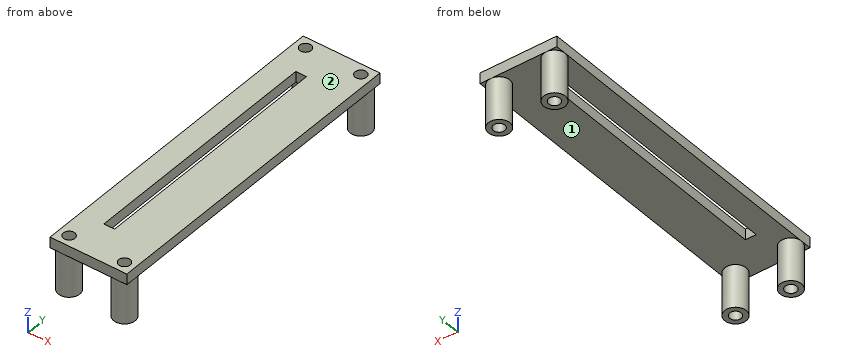
```python
from build123d import *

# Parameters (mm, degrees)
SKETCH1_W           = 21.5
SKETCH1_H           = 91
SKETCH1_R           = 1.6
SKETCH1_W_2         = 3
SKETCH1_H_2         = 69
BOSS_EXTRUDE1_DEPTH = 3
BOSS_EXTRUDE2_START = -12
SKETCH2_R           = 3
SKETCH2_R_2         = 1.6
BOSS_EXTRUDE2_DEPTH = 12


with BuildPart() as part:
    # Sketch1 → Boss-Extrude1 (new body)
    with BuildSketch(Plane.XY):
        with Locations((10.75, 45.5)):
            Rectangle(SKETCH1_W, SKETCH1_H)
        with Locations((3, 88)):
            Circle(SKETCH1_R, mode=Mode.SUBTRACT)
        with Locations((18.5, 88)):
            Circle(SKETCH1_R, mode=Mode.SUBTRACT)
        with Locations((3, 3)):
            Circle(SKETCH1_R, mode=Mode.SUBTRACT)
        with Locations((18.5, 3)):
            Circle(SKETCH1_R, mode=Mode.SUBTRACT)
        with Locations((8, 45.5)):
            Rectangle(SKETCH1_W_2, SKETCH1_H_2, mode=Mode.SUBTRACT)
    extrude(amount=BOSS_EXTRUDE1_DEPTH)

    # Sketch2 → Boss-Extrude2 (add)
    # profile 1 of 4: a face of its own
    with BuildSketch(Plane.XY.offset(BOSS_EXTRUDE2_START)):
        with Locations((3, 3)):
            Circle(SKETCH2_R)
        with Locations((3, 3)):
            Circle(SKETCH2_R_2, mode=Mode.SUBTRACT)
    # profile 2 of 4: a face of its own
    with BuildSketch(Plane.XY.offset(BOSS_EXTRUDE2_START)):
        with Locations((18.5, 3)):
            Circle(SKETCH2_R)
        with Locations((18.5, 3)):
            Circle(SKETCH2_R_2, mode=Mode.SUBTRACT)
    # profile 3 of 4: a face of its own
    with BuildSketch(Plane.XY.offset(BOSS_EXTRUDE2_START)):
        with Locations((18.5, 88)):
            Circle(SKETCH2_R)
        with Locations((18.5, 88)):
            Circle(SKETCH2_R_2, mode=Mode.SUBTRACT)
    # profile 4 of 4: a face of its own
    with BuildSketch(Plane.XY.offset(BOSS_EXTRUDE2_START)):
        with Locations((3, 88)):
            Circle(SKETCH2_R)
        with Locations((3, 88)):
            Circle(SKETCH2_R_2, mode=Mode.SUBTRACT)
    extrude(amount=BOSS_EXTRUDE2_DEPTH)


solid = part.part
```
Geometry: final body of the model. Coordinates: model frame, mm. Face numbers are marked on the shaded views. Coordinates: 2 decimals unless noted, no trailing zeros. Order: outer loops, then holes, each group sorted by start corner. A loop starts at its lowest first (then second) coordinate and runs counter-clockwise, first axis right, second up. Notation, with made-up numbers: (-22.5, 61) -> (24.5, 61) arc R13 ccw to (24.5, 85) -> close; hole circle Ø4 at (76.5, 72). An arc over 180 degrees is marked (long way). Write item = value, one per line.
(1) Cut plane B-B on y = 23. Return loops of the section in (x, z), plus the area to 3 significant figures.
Solved:
outline = (0, 0) -> (6.5, 0) -> (6.5, 3) -> (0, 3) -> close; (9.5, 0) -> (21.5, 0) -> (21.5, 3) -> (9.5, 3) -> close
area = 55.5 mm²
(2) Line query: line 1 (Y direction, x = 18.5, z = -2.75); line 2 (X direction, y = 88, z = -0.25); line 3 (Z direction, x = 15.25, y = 77). Output: solid intervals per line, ascending.
Solved:
line_1 = 0 to 1.4, 4.6 to 6, 85 to 86.4, 89.6 to 91
line_2 = 0 to 1.4, 4.6 to 6, 15.5 to 16.9, 20.1 to 21.5
line_3 = 0 to 3
(3) Cut plane A-A on z = -8.5. Return loops of the section in (x, y).
Solved:
outline = circle Ø6 at (3, 3); circle Ø6 at (3, 88); circle Ø6 at (18.5, 3); circle Ø6 at (18.5, 88); hole circle Ø3.2 at (3, 3); hole circle Ø3.2 at (3, 88); hole circle Ø3.2 at (18.5, 3); hole circle Ø3.2 at (18.5, 88)
(4) Cut plane C-C on x = 13.5. Return loops of the section in (y, z), plus the area to 3 significant figures.
Solved:
outline = (0, 0) -> (91, 0) -> (91, 3) -> (0, 3) -> close
area = 273 mm²
(5) Pull-direction query (Y, two-part tool) for the marked faces 1 and 2; classes: pulls with the +Y half, pulls with the -Y half, needs draft (parallel to the pull), parting line crosses it, or undercut.
Solved:
face_1 = undercut
face_2 = needs draft
(6) Pin query (flat end, axial travel): pin 1 Ø1.9 at (x, y) = (3, 3) entering from +Z; pin 2 Ø11 at (x, y) = (7.5, 32.5) entering from -Z. Return the tip coordinate at first contact, or that it passes through.
Solved:
pin_1 = through
pin_2 = 0
